Input: part model. Units: mm. Frame: model coordinates. A direction names the side the tool comes from. Coordinates: 2 decimals unless noted, no trailing zeros. Loops run counter-clockwise (first coordinate to the right, second up) from the corner with the lowest first, then second, coordinate; pieces in that order, holes last. Notation, with made-up numbers: (76, 61) -> (135, 61) arc R22 cw to (135, 85) -> close; hole circle Ø2 at (63.25, -34). An arc over 180 degrees is marked (long way). Answer as a JSON object with one key per item and string values.
from build123d import *

# Parameters (mm, degrees)
F0_R     = 38.1
F0_R_2   = 3.175
F0_R_3   = 4.826
F1_DEPTH = 15.875
F2_T     = -4.7625
F3_SIZE  = 1.27


with BuildPart() as f1:
    # F0 (on Top) → F1 (new body)
    with BuildSketch(Plane.XY):
        Circle(F0_R)
        with Locations((-30.466994, 0)):
            Circle(F0_R_2, mode=Mode.SUBTRACT)
        Circle(F0_R_3, mode=Mode.SUBTRACT)
        with Locations((30.171195, 0)):
            Circle(F0_R_2, mode=Mode.SUBTRACT)
    extrude(amount=F1_DEPTH)

    # F2
    f2_openings = [f1.faces().sort_by_distance(p)[0] for p in [
        (-37.022369, 0, 15.875),
    ]]
    offset(amount=F2_T, openings=f2_openings)

    # F3
    f3_edges = [f1.edges().sort_by_distance(p)[0] for p in [
        (-38.1, 0, 15.875),
    ]]
    chamfer(f3_edges, length=F3_SIZE)


solid = f1.part
1. Section query B-B (y = 0). Return loops of the section in (x, z) (1 decimal), plus the area to 3 significant figures.
Reply:
{"outline": "(-38.1, 0) -> (-33.6, 0) -> (-33.6, 15.9) -> (-36.8, 15.9) -> (-38.1, 14.6) -> close; (-27.3, 0) -> (-4.8, 0) -> (-4.8, 15.9) -> (-9.6, 15.9) -> (-9.6, 4.8) -> (-22.5, 4.8) -> (-22.5, 15.9) -> (-27.3, 15.9) -> close; (4.8, 0) -> (27, 0) -> (27, 15.9) -> (22.2, 15.9) -> (22.2, 4.8) -> (9.6, 4.8) -> (9.6, 15.9) -> (4.8, 15.9) -> close; (33.3, 0) -> (38.1, 0) -> (38.1, 14.6) -> (36.8, 15.9) -> (33.3, 15.9) -> close", "area": "569 mm2"}
2. Access query for faces 1 (the face through (-27.439, 0.954, 7.826)), 2 (the face through (7, -7, 4.762)). Directions: +Z, -Z, +X, -X, +Y, -Y. A direction counts if a zero-diameter tool reaches every point of the face in a straight line with its end or side. Return the directions, or none.
Reply:
{"face 1": "+Z, -Z", "face 2": "+Z"}
3. Section query A-A (x = 0). Return loops of the section in (y, z) (1 decimal).
Reply:
{"outline": "(-38.1, 0) -> (-4.8, 0) -> (-4.8, 15.9) -> (-9.6, 15.9) -> (-9.6, 4.8) -> (-33.3, 4.8) -> (-33.3, 15.9) -> (-36.8, 15.9) -> (-38.1, 14.6) -> close; (4.8, 0) -> (38.1, 0) -> (38.1, 14.6) -> (36.8, 15.9) -> (33.3, 15.9) -> (33.3, 4.8) -> (9.6, 4.8) -> (9.6, 15.9) -> (4.8, 15.9) -> close"}
4. Line query: line 1 along Y through (x, z) = (24.5, 9); line 2 along Y through (x, z) = (23.5, 9.75); line 3 along X through (y, z) = (8.5, 12.5). Output: solid intervals per line, ascending.
Reply:
{"line 1": "y = -29.18 to -22.61, -5.55 to 5.55, 22.61 to 29.18", "line 2": "y = -29.99 to -23.65, -4.3 to 4.3, 23.65 to 29.99", "line 3": "x = -37.14 to -32.24, -4.44 to 4.44, 32.24 to 37.14"}
5. Pin query (flat end, axial travel): P1, Ø1.5, axis at y = -20.5, z = 8.5, coming from the -X side; P2, Ø2, axis at y = 18, z = 4, coming from the -X side; P3, Ø8, axis at y = -30, z = 9.5, coming from the +X side. Return the tip coordinate at first contact, or that it passes through.
Reply:
{"P1": "stops at x = -32.58", "P2": "stops at x = -34.1", "P3": "stops at x = 27.85"}
6. Section query C-C (z = 9). Count the separate pieces of the cut face and the enclosed holes in it, plus the area to 3 significant figures.
Reply:
{"separate pieces": "2", "enclosed holes": "4", "area": "1,500 mm2"}
7. Mould query, pull axis X, two halves, no side actions, for faces 3 (the face through (4, -4, 15.875)), 4 (the face through (-30.235, -23.183, 7.2)), 5 (the face through (33.2, 0.95, 7.83)). Classes: pulls with the +X half, pulls with the -X half, needs draft (parallel to the pull), parting line crosses it, or undercut.
Reply:
{"face 3": "needs draft", "face 4": "parting line crosses it", "face 5": "undercut"}
